from build123d import *

# Parameters (mm, degrees)
BOSS_EXTRUDE1_DEPTH = 6.35
SKETCH2_R           = 4.7625
CUT_EXTRUDE1_DEPTH  = 153.880572291
CHAMFER1_SIZE       = 2.54


with BuildPart() as part:
    # Sketch1 → Boss-Extrude1 (new body)
    with BuildSketch(Plane(origin=(0, 0, 0), x_dir=(0, 1, 0), z_dir=(0, 0, 1))):
        with BuildLine():
            Line((0, -25.4), (-125.222, -25.4))
            ThreePointArc((-125.222, -25.4), (-150.622, 0), (-125.222, 25.4))
            Line((-125.222, 25.4), (0, 25.4))
            ThreePointArc((0, 25.4), (25.4, 0), (0, -25.4))
        make_face()
    extrude(amount=BOSS_EXTRUDE1_DEPTH)

    # Sketch2 → Cut-Extrude1 (cut, through all)
    with BuildSketch(Plane.XY.offset(6.35)):
        Circle(SKETCH2_R)
        with Locations((0, -125.222)):
            Circle(SKETCH2_R)
    extrude(amount=-CUT_EXTRUDE1_DEPTH, mode=Mode.SUBTRACT)

    # Chamfer1
    chamfer1_edges = [part.edges().sort_by_distance(p)[0] for p in [
        (-4.7625, 0, 0),
        (-4.7625, -125.222, 0),
        (0, 25.4, 0),
        (25.4, -62.611, 0),
        (0, -150.622, 0),
        (-25.4, -62.611, 0),
    ]]
    chamfer(chamfer1_edges, length=CHAMFER1_SIZE)


solid = part.part
The listing builds one solid part. Answer for the finished solid, in the listing's coordinates (mm). Coordinates: 2 decimals unless noted, no trailing zeros. Write each loop counter-clockwise with the first axis right and the second up, starting at its lowest first coordinate (ties: lowest second). Pieces come first, ordered by that corner, then holes. Notation, with made-up numbers: (4, -40) - (15, -40) arc R28 ccw to (15, -21) - close; hole circle Ø3 at (22, -10). An arc over 180 degrees is marked (long way). Put each result on its own line as item: value.
1. Determine the mould class of faces 1 (the face through (0, -61, 0)), 2 (the face through (-0.62, -120.5, 4.47)), 3 (the face through (-0.505, 22.978, 0.123)) for opening direction Y: pulls with the +Y half, pulls with the -Y half, needs draft (parallel to the pull), parting line crosses it, or undercut.
Answer sheet:
face 1: needs draft
face 2: undercut
face 3: pulls with the +Y half
2. The part is cut by section B-B on z = 3.75. Give the vertices of the cut face in (x, y) (1 decimal).
Answer sheet:
outline: (-25.4, -125.2) arc R25.4 ccw to (25.4, -125.2) - (25.4, 0) arc R25.4 ccw to (-25.4, 0) - close; hole circle Ø9.5 at (0, -125.2); hole circle Ø9.5 at (0, 0)
3. The part is cut by section C-C on y = -17.5. Give the vertices of the cut face in (x, z).
Answer sheet:
outline: (-25.4, 2.54) - (-22.86, 0) - (22.86, 0) - (25.4, 2.54) - (25.4, 6.35) - (-25.4, 6.35) - close
4. Flat-ended cylindrical pins translate along their axes: pin 1 Ø12.5 at (x, y) = (0, -125.222) entering from +Z; pin 2 Ø1 at (y, z) = (-50.5, 0.5) entering from +X. Find the tip coordinate at first contact, or state that the pin passes through.
Answer sheet:
pin 1: stops at z = 6.35
pin 2: stops at x = 23.86
5. Find the intervals of material crossed by line 1 along Y through (x, z) = (0, 4.8); line 2 along Y through (x, z) = (2.5, 2.25); line 3 along X through (y, z) = (17, 3.5), in increasing order. Write a range as from..to.
Answer sheet:
line 1: y = -150.62..-129.98, -120.46..-4.76, 4.76..25.4
line 2: y = -150.21..-129.61, -120.83..-4.39, 4.39..24.99
line 3: x = -18.87..18.87
6. The part is cut by section A-A on x = 0. Give the vertices of the cut face in (y, z), plus the area to 3 significant figures.
Answer sheet:
outline: (-150.62, 2.54) - (-148.08, 0) - (-132.52, 0) - (-129.98, 2.54) - (-129.98, 6.35) - (-150.62, 6.35) - close; (-120.46, 2.54) - (-117.92, 0) - (-7.3, 0) - (-4.76, 2.54) - (-4.76, 6.35) - (-120.46, 6.35) - close; (4.76, 2.54) - (7.3, 0) - (22.86, 0) - (25.4, 2.54) - (25.4, 6.35) - (4.76, 6.35) - close
area: 977 mm^2
